Design review of the part built by this model. Coordinates are the model's own, in mm. Give positions to 0.01 mm unless a question says otherwise; leave off trailing zeros. Loops run counter-clockwise (first coordinate to the right, second up) from the corner with the lowest first, then second, coordinate; pieces in that order, holes last. Notation, with made-up numbers: M 63.25,-34.75 L 82.25,-34.75 A17 cw 82.25,-12.75 Z; hole C 21,-31.5 d6. An arc over 180 degrees is marked long. Use a Markdown table: item, result. Add a question column.
(1) Draft analysis for pull direction X (two halves, no side actions). For faces 1 (the face through (43.18, 0, 1)), 2 (the face through (48, 1.5, -1)), 3 (the face through (67.795, 0.021, -50.319)), state which applies: pulls with the +X half, pulls with the -X half, needs draft (parallel to the pull), parting line crosses it, or undercut.
(2) Add section C-C, the plane y = 0.5. Give the boundary of the cut face in (x, z), then the cut area to 3 significant figures.
(3) Add section B-B, the plane x = 59. Give the boundary of the cut face in (y, z), then the cut area to 3 significant figures.
(4) Add section D-D, the plane z = -35. Give the boundary of the cut face in (x, y) (3 decimals), then the cut area to 3 significant figures.
(5) Add section A-A, the plane z = 0. Give the boundary of the cut face in (x, y), then the cut area to 3 significant figures.
(6) For probe 1 along X at (y, z) = (-0.3, 30); probe 2 along Z at (x, y) = (49, 0.55); probe 3 along Z at (x, y) = (55.5, -0.55), list the stretches that pass through material, from the lowest coordinate up.
(7) Insertion check: pin 1 Ø1 at (x, y) = (69.5, 1) entering from -Z. The pin has a flat end and moves straight along its axis. Give the tip position at first contact, or say it passes through.
```python
from build123d import *

# Parameters (mm, degrees)
SKETCH1_W           = 150
SKETCH1_H           = 150
BOSS_EXTRUDE1_DEPTH = 1.5
CUT_EXTRUDE1_DEPTH  = 3
SKETCH3_R           = 1.55
CUT_EXTRUDE2_DEPTH  = 3
CUT_EXTRUDE3_DEPTH  = 3
SKETCH5_R           = 8
CUT_EXTRUDE4_DEPTH  = 3


with BuildPart() as part:
    # Sketch1 → Boss-Extrude1 (new body, symmetric)
    with BuildSketch(Plane(origin=(0, 0, 0), x_dir=(1, 0, 0), z_dir=(0, 1, 0))):
        Rectangle(SKETCH1_W, SKETCH1_H)
    extrude(amount=BOSS_EXTRUDE1_DEPTH, both=True)

    # Sketch2 → Cut-Extrude1 (cut)
    with BuildSketch(Plane(origin=(0, 1.5, 0), x_dir=(1, 0, 0), z_dir=(0, 1, 0))):
        Polygon((50.251262658, 75), (75, 75), (75, 50.251262658), align=None)
        Polygon((-75, 75), (-75, 50.251262658), (-50.251262658, 75), align=None)
        Polygon((-50.251262658, -75), (-75, -75), (-75, -50.251262658), align=None)
        Polygon((75, -75), (75, -50.251262658), (50.251262658, -75), align=None)
    extrude(amount=-CUT_EXTRUDE1_DEPTH, mode=Mode.SUBTRACT)

    # Sketch3 → Cut-Extrude2 (cut)
    with BuildSketch(Plane(origin=(0, 1.5, 0), x_dir=(1, 0, 0), z_dir=(0, 1, 0))):
        with Locations((69.343145751, 50.251262658)):
            Circle(SKETCH3_R)
        with Locations((50.251262658, 69.343145751)):
            Circle(SKETCH3_R)
        with Locations((-69.343145751, 50.251262658)):
            Circle(SKETCH3_R)
        with Locations((-50.251262658, 69.343145751)):
            Circle(SKETCH3_R)
        with Locations((-69.343145751, -50.251262658)):
            Circle(SKETCH3_R)
        with Locations((-50.251262658, -69.343145751)):
            Circle(SKETCH3_R)
        with Locations((69.343145751, -50.251262658)):
            Circle(SKETCH3_R)
        with Locations((50.251262658, -69.343145751)):
            Circle(SKETCH3_R)
    extrude(amount=-CUT_EXTRUDE2_DEPTH, mode=Mode.SUBTRACT)

    # Sketch4 → Cut-Extrude3 (cut)
    with BuildSketch(Plane(origin=(0, 1.5, 0), x_dir=(1, 0, 0), z_dir=(0, 1, 0))):
        Polygon((50.251262658, 75), (-50.251262658, 75), (-75, 50.251262658), (-75, -50.251262658), (-50.251262658, -75), (50.251262658, -75), (43.180194847, -67.928932188), (43.180194847, 67.928932188), align=None)
    extrude(amount=-CUT_EXTRUDE3_DEPTH, mode=Mode.SUBTRACT)

    # Sketch5 → Cut-Extrude4 (cut)
    with BuildSketch(Plane(origin=(0, 1.5, 0), x_dir=(1, 0, 0), z_dir=(0, 1, 0))):
        with Locations((59, 0)):
            Circle(SKETCH5_R)
        with Locations((59, 30)):
            Circle(SKETCH5_R)
        with Locations((59, -30)):
            Circle(SKETCH5_R)
    extrude(amount=-CUT_EXTRUDE4_DEPTH, mode=Mode.SUBTRACT)


solid = part.part
```
Established:
| question | item | result |
|---|---|---|
| 1 | face 1 | pulls with the -X half |
| 1 | face 2 | needs draft |
| 1 | face 3 | undercut |
| 2 | outline | M 43.18,-67.93 L 50.25,-75 L 75,-50.25 L 75,50.25 L 50.25,75 L 43.18,67.93 Z; hole C 50.25,-69.34 d3.1; hole C 50.25,69.34 d3.1; hole C 59,-30 d16; hole C 59,0 d16; hole C 59,30 d16; hole C 69.34,-50.25 d3.1; hole C 69.34,50.25 d3.1 |
| 2 | area | 3,480 mm^2 |
| 3 | outline | M -1.5,-66.25 L 1.5,-66.25 L 1.5,-38 L -1.5,-38 Z; M -1.5,-22 L 1.5,-22 L 1.5,-8 L -1.5,-8 Z; M -1.5,8 L 1.5,8 L 1.5,22 L -1.5,22 Z; M -1.5,38 L 1.5,38 L 1.5,66.25 L -1.5,66.25 Z |
| 3 | area | 254 mm^2 |
| 4 | outline | M 43.18,-1.5 L 52.755,-1.5 L 52.755,1.5 L 43.18,1.5 Z; M 65.245,-1.5 L 75,-1.5 L 75,1.5 L 65.245,1.5 Z |
| 4 | area | 58.0 mm^2 |
| 5 | outline | M 43.18,-1.5 L 51,-1.5 L 51,1.5 L 43.18,1.5 Z; M 67,-1.5 L 75,-1.5 L 75,1.5 L 67,1.5 Z |
| 5 | area | 47.5 mm^2 |
| 6 | probe 1 | 43.18 to 51, 67 to 75 |
| 6 | probe 2 | -73.75 to -70.26, -68.43 to 68.43, 70.26 to 73.75 |
| 6 | probe 3 | -69.75 to -37.19, -22.81 to -7.19, 7.19 to 22.81, 37.19 to 69.75 |
| 7 | pin 1 | z = -56.25 |
